Autodesk Inventor part; units mm, degrees
ref_plane "YZ Plane" through (0, 0, 0) normal (1, 0, 0) x (0, 1, 0)
ref_plane "XZ Plane" through (0, 0, 0) normal (0, 1, 0) x (-1, 0, 0)
ref_plane "XY Plane" through (0, 0, 0) normal (0, 0, 1) x (1, 0, 0)
sketch "Sketch1" plane through (0, 0, 0) normal (0, 0, 1) x (1, 0, 0)
  line L0 (0, 0) -> (62, 0)
  line L1 (62, 0) -> (62, 12)
  line L2 (58, 16) -> (4, 16)
  line L3 (0, 12) -> (0, 0)
  arc A0 (4, 16) -> (0, 12) centre (4, 12) ccw
  arc A1 (62, 12) -> (58, 16) centre (58, 12) ccw
  point P0 (0, 16)
  dimension "d0" = 16
  dimension "d1" = 62
  dimension "d2" = 4
extrude "Extrusion1" add sketch "Sketch1" along normal blind 57.7
sketch "Sketch2" plane through (0, 0, 0) normal (0, -1, 0) x (1, 0, 0)
  line L0 (62, 0) -> (62, 57.7)
  line L1 (62, 28.85) -> (0, 28.85) construction
  line L2 (0, 0) -> (0, 57.7)
  circle A0 centre (31, 28.85) radius 22.5 construction
  circle A1 centre (53.5, 28.85) radius 2
  circle A2 centre (8.5, 28.85) radius 2
  circle A3 centre (31, 28.85) radius 7.5 construction
  circle A4 centre (38.5, 28.85) radius 2
  circle A5 centre (23.5, 28.85) radius 2
  dimension "d5" = 45
  dimension "d8" = 4
  dimension "d9" = 15
extrude "Extrusion2" cut sketch "Sketch2" against normal through all
properties part number "4aa-holder"
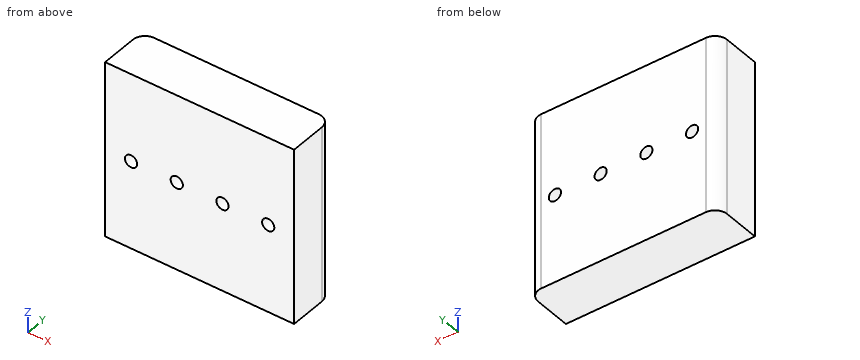
Design review of the part built by this model. Coordinates are the model's own, in mm. Round coordinates to 2 decimals unless told otherwise and drop trailing zeros. Write each loop counter-clockwise with the first axis right and the second up, starting at its lowest first coordinate (ties: lowest second). Pieces come first, ordered by that corner, then holes. Notation, with made-up numbers: (32.5, 70) -> (61.5, 70) arc R22 cw to (61.5, 103) -> close; hole circle Ø9 at (-22, 59.25). An arc over 180 degrees is marked (long way). One line per item, written item: value. Start each with the question number.
Q1. Add section B-B (x = 53.5). Give the boundary of the cut face in (y, z), then the cut area to 3 significant figures.
Q2. Add section C-C (y = 14.5). Give the boundary of the cut face in (x, z), then the cut area to 3 significant figures.
Q3. To check wall thickness, follow probe 1 along Z at (x, y) = (38.5, 3.5); probe 2 along Z at (x, y) = (37.5, 9.25); probe 3 along X at (y, z) = (14, 16). State the ranges of each line that lie inside material, in increasing order.
Q4. Add section A-A (z = 28.85). Give the boundary of the cut face in (x, y), then the cut area to 3 significant figures.
Q5. Insertion check: P1, Ø3.5, axis at x = 8.5, z = 28.85, coming from the -Y side. The pin has a flat end and moves straight along its axis. Give the tip position at first contact, or say it passes through.
Response:
1. outline: (0, 0) -> (16, 0) -> (16, 26.85) -> (0, 26.85) -> close; (0, 30.85) -> (16, 30.85) -> (16, 57.7) -> (0, 57.7) -> close
1. area: 859 mm^2
2. outline: (0.88, 0) -> (61.12, 0) -> (61.12, 57.7) -> (0.88, 57.7) -> close; hole circle Ø4 at (8.5, 28.85); hole circle Ø4 at (23.5, 28.85); hole circle Ø4 at (38.5, 28.85); hole circle Ø4 at (53.5, 28.85)
2. area: 3,430 mm^2
3. probe 1: z = 0 to 26.85, 30.85 to 57.7
3. probe 2: z = 0 to 27.12, 30.58 to 57.7
3. probe 3: x = 0.54 to 61.46
4. outline: (0, 0) -> (6.5, 0) -> (6.5, 16) -> (4, 16) arc R4 ccw to (0, 12) -> close; (10.5, 0) -> (21.5, 0) -> (21.5, 16) -> (10.5, 16) -> close; (25.5, 0) -> (36.5, 0) -> (36.5, 16) -> (25.5, 16) -> close; (40.5, 0) -> (51.5, 0) -> (51.5, 16) -> (40.5, 16) -> close; (55.5, 0) -> (62, 0) -> (62, 12) arc R4 ccw to (58, 16) -> (55.5, 16) -> close
4. area: 729 mm^2
5. P1: passes through
